Solid Edge part; units mm, degrees
sketch "Sketch1" plane through (0, 0, 0) normal (1, 0, 0) x (0, 1, 0)
  line L0 (150, 300) -> (0, 150)
  line L1 (0, 150) -> (0, 0)
  line L2 (0, 0) -> (350, 0)
  line L3 (350, 0) -> (350, 300)
  line L4 (350, 300) -> (150, 300)
extrude "Protrusion1" add sketch "Sketch1" against normal blind 15
sketch "Sketch2" plane through (-10, 350, 150) normal (0, 1, 0) x (0, 0, -1)
  line L0 (-150, 442) -> (-150, -10)
  line L1 (-150, -10) -> (150, -10)
  line L2 (150, -10) -> (150, 442)
  line L3 (150, 442) -> (-150, 442)
extrude "ProtrusiónExtruida_3" add sketch "Sketch2" along normal blind 15
sketch "Sketch3" plane through (-452, 360, 150) normal (-1, 0, 0) x (0, 0, 1)
  line L0 (150, -210) -> (0, -360)
  line L1 (0, -360) -> (-150, -360)
  line L2 (-150, -360) -> (-150, -10)
  line L3 (-150, -10) -> (150, -10)
  line L4 (150, -10) -> (150, -210)
extrude "ProtrusiónExtruida_5" add sketch "Sketch3" against normal blind 15
sketch "Sketch4" plane through (-226, 185, 0) normal (0, 0, -1) x (1, 0, 0)
  line L0 (-226, 185) -> (226, 185)
  line L1 (226, 185) -> (226, -180)
  line L2 (226, -180) -> (-226, -180)
  line L3 (-226, -180) -> (-226, 185)
extrude "ProtrusiónExtruida_6" add sketch "Sketch4" along normal blind 10
fillet "Redondeo_5" radius 20 2 edges at (-7.5, 150, 300) (-444.5, 150, 300)
sketch "Sketch5" plane through (-226, 175, 0) normal (0, 0, 1) x (1, 0, 0)
  line L0 (-211, -6.7157) -> (211, -6.7157)
  line L1 (211, -6.7157) -> (211, -16.7157)
  line L2 (-211, -16.7157) -> (211, -16.7157)
  line L3 (-211, -16.7157) -> (-211, -6.7157)
  line L4 (-211, -56.7157) -> (211, -56.7157)
  line L5 (211, -46.7157) -> (211, -56.7157)
  line L6 (-211, -46.7157) -> (211, -46.7157)
  line L7 (-211, -56.7157) -> (-211, -46.7157)
extrude "ProtrusiónExtruida_12" add sketch "Sketch5" along normal blind 300
fillet "Redondeo_13" radius 10 6 edges at (-226, 118.2843, 0) (-226, 168.2843, 0) (-437, 0, 75) (-15, 0, 75) (-437, 168.2843, 150) (-15, 168.2843, 150)
sketch "Sketch6" plane through (-437, 123.2843, 284.1421) normal (-1, 0, 0) x (0, -1, 0)
  line L0 (15.8227, 25.3838) -> (15.8227, -26.6806)
  line L1 (-10.8579, 25.3838) -> (15.8227, 25.3838)
  line L2 (-10.8579, 0) -> (-10.8579, 25.3838)
  line L3 (-10.8579, 0) -> (15.8227, -26.6806)
extrude "VaciadoExtruido_1" cut sketch "Sketch6" against normal blind 516.6501
fillet "Round1" radius 10 8 edges at (-437, 118.2843, 139.1421) (-437, 115.3553, 2.9289) (-437, 59.1421, 0) (-439.9289, 2.9289, 0) (-15, 118.2843, 139.1421) (-15, 115.3553, 2.9289) (-15, 59.1421, 0) (-12.0711, 2.9289, 0)
hole "Agujero_3" at (-342.6083, 118.2843, 137.5113) direction (0, 1, 0) diameter 50 end up to next
hole "Agujero_4" at (-182.6083, 168.2843, 137.5113) direction (0, -1, 0) diameter 50 end up to next
Part model, mm, in its own coordinate system. A direction names the side the tool comes from. Round coordinates to 2 decimals unless told otherwise and drop trailing zeros. Write each loop counter-clockwise with the first axis right and the second up, starting at its lowest first coordinate (ties: lowest second). Pieces come first, ordered by that corner, then holes. Notation, with made-up numbers: M 25.25,33 L 67.25,33 A33 cw 67.25,70 Z; hole C 25,42.25 d5. An arc over 180 degrees is marked long. Return JSON: item names as keys, results as strings. Group by question number.
(1) Saw through at D-D on x = -352.5. Write the cut outline in (y, z).
(2) Saw through at B-B on x = -404.5. Write the cut outline in (y, z).
(3) Two-plate mould, pull along Y, no slides. Class faces 1 (the face through (-15, 263, 148)), 2 (the face through (-444.4, 150.73, 298.52)), 3 (the face through (-15, 58, 105)): +Y half, -Y half, draft (parallel to the pull), parting line (faces both ways), or undercut.
(4) Which spindle directions (+Z, -Z, +X, -X, +Y, -Y) get a long thin tool onto all of the face, cutting with end or side? Do faces 4 (the face through (-317.82, 123.21, 140.77)), 5 (the face through (-229, 158.284, 148)), 6 (the face through (-433.993, 115.433, 140.95)). Say none if no direction does.
(5) Saw through at A-A on z = 30. Write the cut outline in (x, y), then the cut area to 3 significant figures.
(6) Drill centre lines: probe 1 along Y at (x, z) = (-185, 210.5); probe 2 along X at (y, z) = (259, 278); probe 3 along Y at (x, z) = (-20.5, 73.5). Where is each one in solid material? Low to high.
(7) Pin check, flat tip, straight feed: pin 1 Ø1.5 at (x, z) = (-406, 150) entering from -Y. Stop position of the tip, or through.
(8) Saw through at C-C on y = 90.5. Write the cut outline in (x, z), then the cut area to 3 significant figures.
Returned:
{
 "1": {"outline": "M 0,-10 L 365,-10 L 365,300 L 350,300 L 350,0 L 178.28,0 A10 cw 168.28,10 L 168.28,300 L 158.28,300 L 158.28,0 L 128.28,0 L 128.28,114.55 L 118.28,114.55 L 118.28,10 A10 cw 108.28,0 L 0,0 Z; M 118.28,160.47 L 128.28,160.47 L 128.28,278.28 L 118.28,268.28 Z"},
 "2": {"outline": "M 0,-10 L 365,-10 L 365,300 L 350,300 L 350,0 L 178.28,0 A10 cw 168.28,10 L 168.28,300 L 158.28,300 L 158.28,0 L 128.28,0 L 128.28,278.28 L 118.28,268.28 L 118.28,10 A10 cw 108.28,0 L 0,0 Z"},
 "3": {"face 1": "undercut", "face 2": "-Y half", "face 3": "draft"},
 "4": {"face 4": "-Y", "face 5": "+Z", "face 6": "+Z, -Y"},
 "5": {"outline": "M -452,0 L -447,0 A10 ccw -437,10 L -437,108.28 A10 cw -427,118.28 L -25,118.28 A10 cw -15,108.28 L -15,10 A10 ccw -5,0 L 0,0 L 0,365 L -452,365 Z; hole M -437,128.28 L -15,128.28 L -15,158.28 L -437,158.28 Z; hole M -437,178.28 A10 ccw -427,168.28 L -25,168.28 A10 ccw -15,178.28 L -15,350 L -437,350 Z", "area": "25,800 mm²"},
 "6": {"probe 1": "118.28 to 128.28, 158.28 to 168.28, 350 to 365", "probe 2": "-452 to -437, -15 to 0", "probe 3": "117.21 to 128.28, 158.28 to 169.35, 350 to 365"},
 "7": {"pin 1": "y = 118.28"},
 "8": {"outline": "M -452,-10 L 0,-10 L 0,240.5 L -15,240.5 L -15,10 A10 cw -25,0 L -427,0 A10 cw -437,10 L -437,240.5 L -452,240.5 Z", "area": "11,800 mm²"}
}
